from build123d import *

# Parameters (mm, degrees)
F1_DEPTH = 31
F6_DEPTH = 138
F9_DEPTH = 188


with BuildPart() as f1:
    # F0 (on Right) → F1 (new body)
    with BuildSketch(Plane.YZ):
        Polygon((38.1051177665, 66), (-38.1051177665, 66), (-76.210235533, 0), (-38.1051177665, -66), (38.1051177665, -66), (76.210235533, 0), align=None)
    extrude(amount=F1_DEPTH)

    # F2 (on Front) → F3 (revolve)
    with BuildSketch(Plane.XZ):
        with BuildLine():
            Line((31, 0), (141, 0))
            ThreePointArc((141, 0), (114.7994974843, 52.6497863244), (57, 63.4980314656))
            ThreePointArc((57, 63.4980314656), (43.1856174465, 57.8259895094), (31, 49.193495505))
            Line((31, 49.193495505), (31, 0))
        make_face()
    revolve(axis=Axis((75, 0, 0), (-1, 0, 0)))

    # F5 (on offset) → F6 (cut)
    with BuildSketch(Plane(origin=(0, 0, -66), x_dir=(1, 0, 0), z_dir=(0, 0, -1))):
        with BuildLine():
            Line((57, -20), (137.8967407741, -20))
            ThreePointArc((137.8967407741, -20), (140.0304895149, 11.2709996651), (127.4976189936, 40))
            Line((127.4976189936, 40), (75, 40))
            Line((75, 40), (57, 40))
            Line((57, 40), (57, 0))
            Line((57, 0), (57, -20))
        make_face()
    extrude(amount=-F6_DEPTH, mode=Mode.SUBTRACT)

    # F8 (on offset) → F9 (cut)
    with BuildSketch(Plane(origin=(0, 0, -66), x_dir=(1, 0, 0), z_dir=(0, 0, -1))):
        with BuildLine():
            Line((90, -20), (110.5558559129, -55.6037868342))
            ThreePointArc((110.5558559129, -55.6037868342), (127.3463070124, -40.197812654), (137.8967407741, -20))
            Line((137.8967407741, -20), (90, -20))
        make_face()
    extrude(amount=-F9_DEPTH, mode=Mode.SUBTRACT)


solid = f1.part
Model file for the job. Use its own axes, mm. A direction names the side the tool comes from. Give positions to 0.01 mm unless a question says otherwise; leave off trailing zeros. Loops run counter-clockwise (first coordinate to the right, second up) from the corner with the lowest first, then second, coordinate; pieces in that order, holes last.
1) Saw through at C-C (x = 19). Write the cut outline in (y, z).
2) Wall check: line 1 (X direction, y = -13.5, z = 35.5); line 2 (X direction, y = 50, z = 25.5); line 3 (Y direction, x = 97, z = 12.5). Give the ranges that are in metal, low to high.
3) Pull direction Y, two halves, no side cores. Call faces 4 (the flat face through (57, -10, -1)), 5 (the flat face through (15.283, 57.424, 32.538)), 6 (the flat face through (85, -40, -1)), 7 (the flat face through (15.283, -57.424, -32.538)): +Y half, -Y half, draft (parallel to the pull), parting line (faces both ways), or undercut.
4) Saw through at A-A (y = -55.5). Write the cut outline in (x, z).
5) Tool access for faces 1 (the flat face through (31, 50, 1)), 2 (the flat face through (97.85, 33.6, -0.86)), 3 (the flat face through (0, -1, 1)): list every direction of +Z, -Z, +X, -X, +Y, -Y with a clear straight run to the whole face (end or side of a thin tool).
6) Saw through at D-D (y = -5). Write the cut outline in (x, z), plus the area to 3 significant figures.
7) Saw through at B-B (z = -40). Write the cut outline in (x, y).
8) Flat gauge pins, fed straight in: pin 1 Ø1.5 at (x, y) = (72.5, 37) entering from -Z; pin 2 Ø4 at (y, z) = (-41.5, -31.5) entering from +X; pin 3 Ø3 at (y, z) = (-58.5, -12.5) entering from +X; pin 4 Ø5 at (y, z) = (-34, -45.5) entering from -X. Where does each tip first touch, or does it go through?
Answer block:
1. outline: (-76.21, 0) - (-38.11, -66) - (38.11, -66) - (76.21, 0) - (38.11, 66) - (-38.11, 66) - close
2. line 1: x = 0 to 57
2. line 2: x = 0 to 31, 40.28 to 107.32
2. line 3: y = -60.96 to -40, 32.12 to 60.96
3. face 4: undercut
3. face 5: +Y half
3. face 6: undercut
3. face 7: -Y half
4. outline: (0, -35.87) - (31, -35.87) - (31, 35.87) - (0, 35.87) - close; circle Ø71.44 at (75, 0)
5. face 1: none
5. face 2: +Z, -Z, +X
5. face 3: +Z, -Z, -X, +Y, -Y
6. outline: (0, -66) - (31, -66) - (31, -48.94) arc R65.81 ccw to (57, -63.3) - (57, 63.3) arc R65.81 ccw to (31, 48.94) - (31, 66) - (0, 66) - close
6. area: 7,080 mm2
7. outline: (0, -53.12) - (31, -53.12) - (31, -28.64) arc R52.5 ccw to (109, -40) - (57, -40) - (57, 20) - (90, 20) - (103.8, 43.9) arc R52.5 ccw to (31, 28.64) - (31, 53.12) - (0, 53.12) - close
8. pin 1: stops at z = -55.1
8. pin 2: stops at x = 117.96
8. pin 3: stops at x = 105.9
8. pin 4: stops at x = 0
